Print and shaded views of the part. All mm, measured from the part's lowest x, y and z. Round coordinates to 2 decimals unless told otherwise and drop trailing zeros. Order: outer loops, then holes, each group sorted by start corner. A loop starts at its lowest first (then second) coordinate and runs counter-clockwise, first axis right, second up. Notation, with made-up numbers: (34.5, 12) - (39.5, 12) arc R11 ccw to (39.5, 18) - close; hole circle Ø2 at (80, 18.5). An arc over 180 degrees is marked (long way). Return JSON: item names as keys, results as strings. Group by question number.
Item 1: Saw through at C-C on x = 3.25. List the corners of the cut face in (y, z), and give its area (3 significant figures).
Item 2: Saw through at B-B on z = 38.5. List the corners of the cut face in (x, y) (3 decimals).
Item 3: Two-plate mould, pull along Y, no slides. Class the marked faces 1 and 2: released by +Y, released by -Y, zero draft, split by the parting line, or undercut.
Item 4: Probe probe 1 along X at (y, z) = (0.4, 34) (3 decimals); probe 2 along Z at (x, y) = (2.25, 2.6). List the from-to ranges inside material, lowest first.
Item 5: Drop flat-ended pins along their axis: pin 1 (1.5 mm diameter, centred on y = 2, z = 5.5, fed in from -X); pin 2 (0.9 mm diameter, centred on x = 1.5, y = 1, fed in from +Z). Give the stop position or say it passes through.
Item 6: Saw through at A-A on y = 0.55. List the corners of the cut face in (x, z) (3 decimals), and give its area (3 significant figures).
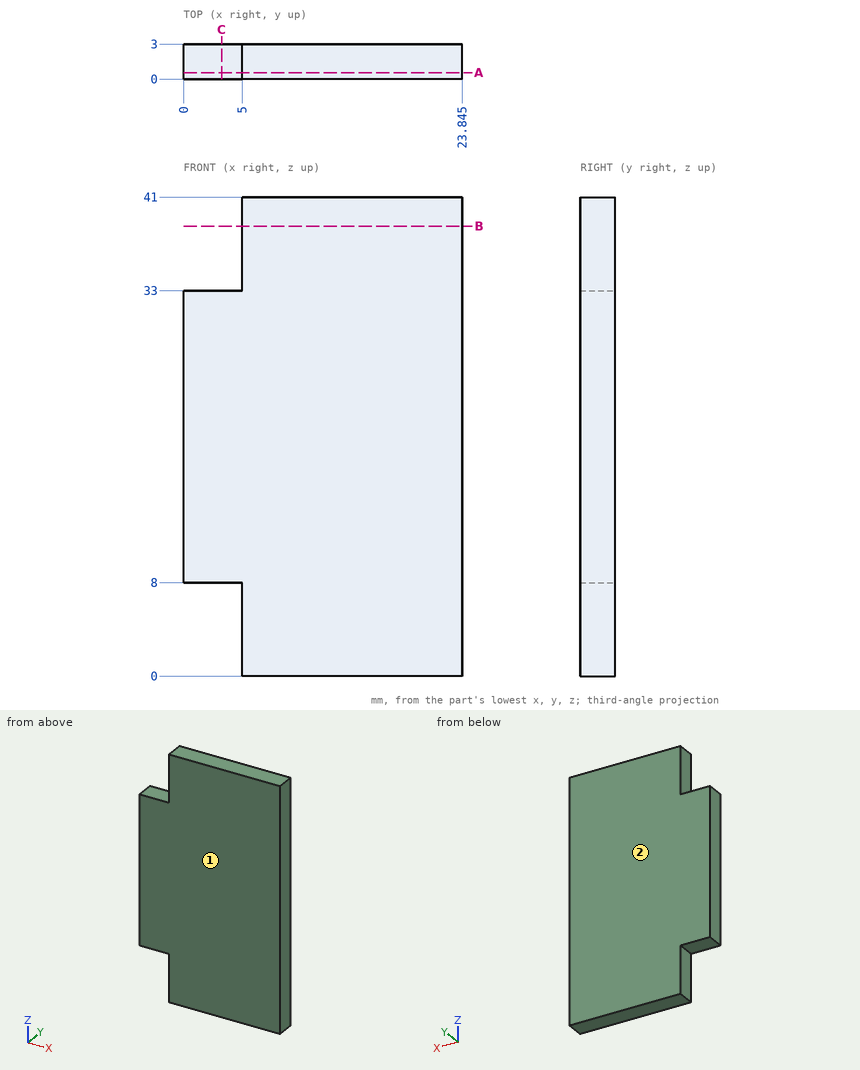
Filled in:
{
 "1": {"outline": "(0, 8) - (3, 8) - (3, 33) - (0, 33) - close", "area": "75.0 mm^2"},
 "2": {"outline": "(5, 0) - (23.845, 0) - (23.845, 3) - (5, 3) - close"},
 "3": {"face 1": "released by -Y", "face 2": "released by +Y"},
 "4": {"probe 1": "x = 5 to 23.845", "probe 2": "z = 8 to 33"},
 "5": {"pin 1": "stops at x = 5", "pin 2": "stops at z = 33"},
 "6": {"outline": "(0, 8) - (5, 8) - (5, 0) - (23.845, 0) - (23.845, 41) - (5, 41) - (5, 33) - (0, 33) - close", "area": "898 mm^2"}
}
